from build123d import *

# Parameters (mm, degrees)
F0_W     = 160
F0_H     = 250
F1_DEPTH = 8
F2_R     = 35
F2_R_2   = 1.6
F2_R_3   = 12.5
F3_DEPTH = 8.001
F4_R     = 5
F5_DEPTH = 8.001
F6_R     = 50


with BuildPart() as f1:
    # F0 (on Top) → F1 (new body)
    with BuildSketch(Plane.XY):
        with Locations((0, -45)):
            Rectangle(F0_W, F0_H)
    extrude(amount=F1_DEPTH)

    # F2 (on Top) → F3 (cut, through all)
    with BuildSketch(Plane.XY):
        Circle(F2_R)
        with Locations((-15.5, 69.5)):
            Circle(F2_R_2)
        with Locations((15.5, 69.5)):
            Circle(F2_R_2)
        with Locations((15.5, 38.5)):
            Circle(F2_R_2)
        with Locations((-15.5, 38.5)):
            Circle(F2_R_2)
        with Locations((0, 54)):
            Circle(F2_R_3)
        with Locations((-67.938766, 21.326606)):
            Circle(F2_R_2)
        with Locations((-41.091978, 5.826606)):
            Circle(F2_R_2)
        with Locations((-25.591978, 32.673394)):
            Circle(F2_R_2)
        with Locations((-52.438766, 48.173394)):
            Circle(F2_R_2)
        with Locations((-46.765372, 27)):
            Circle(F2_R_3)
        with Locations((-52.438766, -48.173394)):
            Circle(F2_R_2)
        with Locations((-25.591978, -32.673394)):
            Circle(F2_R_2)
        with Locations((-41.091978, -5.826606)):
            Circle(F2_R_2)
        with Locations((-67.938766, -21.326606)):
            Circle(F2_R_2)
        with Locations((-46.765372, -27)):
            Circle(F2_R_3)
        with Locations((15.5, -69.5)):
            Circle(F2_R_2)
        with Locations((15.5, -38.5)):
            Circle(F2_R_2)
        with Locations((-15.5, -38.5)):
            Circle(F2_R_2)
        with Locations((-15.5, -69.5)):
            Circle(F2_R_2)
        with Locations((0, -54)):
            Circle(F2_R_3)
        with Locations((67.938766, -21.326606)):
            Circle(F2_R_2)
        with Locations((41.091978, -5.826606)):
            Circle(F2_R_2)
        with Locations((25.591978, -32.673394)):
            Circle(F2_R_2)
        with Locations((52.438766, -48.173394)):
            Circle(F2_R_2)
        with Locations((46.765372, -27)):
            Circle(F2_R_3)
        with Locations((52.438766, 48.173394)):
            Circle(F2_R_2)
        with Locations((25.591978, 32.673394)):
            Circle(F2_R_2)
        with Locations((41.091978, 5.826606)):
            Circle(F2_R_2)
        with Locations((67.938766, 21.326606)):
            Circle(F2_R_2)
        with Locations((46.765372, 27)):
            Circle(F2_R_3)
    extrude(amount=F3_DEPTH, mode=Mode.SUBTRACT)

    # F4 (on Top) → F5 (cut, through all)
    with BuildSketch(Plane.XY):
        with Locations((57.275649, 57.275649)):
            Circle(F4_R)
        with Locations((-57.275649, 57.275649)):
            Circle(F4_R)
        with Locations((-57.275649, -57.275649)):
            Circle(F4_R)
        with Locations((57.275649, -57.275649)):
            Circle(F4_R)
    extrude(amount=F5_DEPTH, mode=Mode.SUBTRACT)

    # F6
    f6_edges = [f1.edges().sort_by_distance(p)[0] for p in [
        (80, 80, 4),
        (-80, 80, 4),
    ]]
    fillet(f6_edges, radius=F6_R)


solid = f1.part
Read the model definition and answer for the solid it produces. Units are mm, in the model's axes. Coordinates: 2 decimals unless noted, no trailing zeros. Order: outer loops, then holes, each group sorted by start corner. A loop starts at its lowest first (then second) coordinate and runs counter-clockwise, first axis right, second up. Notation, with made-up numbers: (77, 5.5) - (102, 5.5) arc R16 ccw to (102, 16.5) - close; hole circle Ø8 at (80.25, -20). An arc over 180 degrees is marked (long way). Use one line per item in the form item = value.
(1) Given pin 1 Ø3 at (x, z) = (46, 5) entering from +Y, flat-ended and moving along its own axis, determine where the tip first touches the part or whether it passes through.
Computed values:
pin_1 = 77.85
(2) Section B-B, the plane y = -27 is taken. Give the vertices of the cut face in (x, z), then the cut area to 3 significant figures.
Computed values:
outline = (-80, 0) - (-59.27, 0) - (-59.27, 8) - (-80, 8) - close; (-34.27, 0) - (-22.27, 0) - (-22.27, 8) - (-34.27, 8) - close; (22.27, 0) - (34.27, 0) - (34.27, 8) - (22.27, 8) - close; (59.27, 0) - (80, 0) - (80, 8) - (59.27, 8) - close
area = 524 mm²
(3) Section A-A, the plane x = 0 is taken. Give the vertices of the cut face in (y, z).
Computed values:
outline = (-170, 0) - (-66.5, 0) - (-66.5, 8) - (-170, 8) - close; (-41.5, 0) - (-35, 0) - (-35, 8) - (-41.5, 8) - close; (35, 0) - (41.5, 0) - (41.5, 8) - (35, 8) - close; (66.5, 0) - (80, 0) - (80, 8) - (66.5, 8) - close
(4) For a pull along X with two mould halves and no side action, classify faces 1 (the face through (-1, -170, 4)), 2 (the face through (64.964, 65.742, 4.056)), 3 (the face through (-80, -71, 4)), 4 (the face through (-57.93, -52.32, 3.94)) as pulls with the +X half, pulls with the -X half, needs draft (parallel to the pull), parting line crosses it, or undercut.
Computed values:
face_1 = needs draft
face_2 = pulls with the +X half
face_3 = pulls with the -X half
face_4 = undercut
(5) Straight lines are drawn through the part: L1, parallel to X at y = -69.5, z = 2.5; L2, parallel to Y at x = 16.5, z = 4; L3, parallel to X at y = 26.5, z = 1. For each, find the intervals that lie inside material, in ascending order.
Computed values:
L1 = -80 to -17.1, -13.9 to 13.9, 17.1 to 80
L2 = -170 to -70.75, -68.25 to -39.75, -37.25 to -30.87, 30.87 to 37.25, 39.75 to 68.25, 70.75 to 80
L3 = -80 to -59.26, -34.28 to -22.86, 22.86 to 34.28, 59.26 to 80
(6) Section C-C, the plane z = 5.75 is taken. Give the number of separate pieces and of enclosed holes in the cut face, then the cut area to 3 significant figures.
Computed values:
separate_pieces = 1
enclosed_holes = 35
area = 31,600 mm²
